Autodesk Fusion 360 part; units mm, degrees
sketch "Sketch1" plane through (0, 0, 0) normal (0, 1, 0) x (1, 0, 0)
  line L0 (0, 0) -> (0, -1175.3412)
  line L1 (0, -1175.3412) -> (0, 325) construction
  line L2 (0, 0) -> (-1356.5029, 0) construction
  circle A0 centre (871.6879, -79.2241) radius 125
  circle A1 centre (871.6879, -79.2241) radius 250
  line L3 (-50, 255) -> (50, 255)
  line L4 (50, 321.1308) -> (50, 933.0127)
  line L5 (-50, 945) -> (-50, 255)
  line L6 (250, 433.0127) -> (250, 933.0127)
  line L7 (-250, 933.0127) -> (-250, 433.0127)
  line L8 (635.6485, 3.1495) -> (499.9901, 3.1495)
  line L9 (490.5883, -96.5563) -> (622.2894, -96.5563)
  line L10 (-1356.5029, 0) -> (466.5356, 0) construction
  line L11 (634.5728, 0) -> (675.4964, 0) construction
  line L12 (775, 0) -> (1559.7574, 0) construction
  line L13 (250, 933.0127) -> (48.2627, 933.0127)
  line L14 (-48.2627, 933.0127) -> (-250, 933.0127)
  line L15 (-48.2627, 933.0127) -> (-50, 945) construction
  arc A2 (-250, 433.0127) -> (250, 433.0127) centre (0, 0) ccw
  arc A3 (-50, 321.1308) -> (50, 321.1308) centre (0, 0) ccw
  line L16 (99.0099, -490.099) -> (909.823, -326.2984)
  dimension "d1" = 650
  dimension "d2" = 1000
  dimension "d3" = 250
  dimension "d4" = 500
  dimension "d7" = 500
  dimension "d8" = 500
  dimension "d9" = 933.0127
extrude "Extrude1" add sketch "Sketch1" along normal mid plane 400 contours L0 L4 L6 L13 A2 A3 | L0 L5 L7 L14 A2 A3 | A1 L8 L9 A2 | A1
extrude "Extrude2" add sketch "Sketch1" along normal mid plane 100 contours A1 L9 A2 L16
hole "Hole1" at (250, 0, -683.0127) direction (-1, 0, 0) diameter 200 end through all
Geometry check sheet. Reference: the model listing, model coordinates, mm. A direction names the side the tool comes from. Round coordinates to 2 decimals unless told otherwise and drop trailing zeros. Loops run counter-clockwise (first coordinate to the right, second up) from the corner with the lowest first, then second, coordinate; pieces in that order, holes last.
Item 1: Cross-section at D-D on z = -764. Record the boundary of the cut face in (x, y), then the cut area to 3 significant figures.
Item 2: Cross-section at C-C on x = 545. Record the boundary of the cut face in (y, z), then the cut area to 3 significant figures.
Item 3: Cross-section at B-B on z = -559.5. Record the boundary of the cut face in (x, y).
Item 4: Mould release check, pull along Z, two halves, no side actions. Record for faces 1 (the cylindrical face through (1083.36, -2.8, -53.8)), 2 (the cylindrical face through (430.38, -2.8, -254.505)), 3 (the cylindrical face through (-151.4, -4.4, -583.11)): pulls with the +Z half, pulls with the -Z half, needs draft (parallel to the pull), parting line crosses it, or undercut.
Item 5: Cross-section at A-A on y = 0. Record the boundary of the cut face in (x, z), then the cut area to 3 significant figures.
Item 6: Access from +Z, -Z, +X, -X, +Y, -Y to the whole of each face (thin tool, end or side, straight path). Record for faces 4 (the flat face through (556, -126, 96.556)), 5 (the flat face through (569, -3, -3.15)), 6 (the flat face through (556, 124, 96.556)), 7 (the flat face through (250, -92, -735)).
Item 7: Thickness scan on line 1 (X direction, y = 136, z = 4.5); line 2 (Z direction, x = -144, y = 0); line 3 (X direction, y = -144, z = -685.5). Record the ranges inside material, lowest first.
Item 8: Gauge pin test, flat ends, axial feed: pin 1 (12 mm diameter, centred on x = 737.5, y = 114.5, fed in from -Z); pin 2 (12 mm diameter, centred on x = 521, y = 38, fed in from -Z); pin 3 (8 mm diameter, centred on x = 953, y = 98.5, fed in from -Z). Record the tip position at first contact, or that the pin passes through.
Answer sheet:
1. outline: (-250, -200) - (-50, -200) - (-50, -58.66) - (-250, -58.66) - close; (-250, 58.66) - (-50, 58.66) - (-50, 200) - (-250, 200) - close; (50, -200) - (250, -200) - (250, -58.66) - (50, -58.66) - close; (50, 58.66) - (250, 58.66) - (250, 200) - (50, 200) - close
1. area: 113,000 mm2
2. outline: (-200, -3.15) - (200, -3.15) - (200, 96.56) - (50, 96.56) - (50, 400) - (-50, 400) - (-50, 96.56) - (-200, 96.56) - close
2. area: 70,200 mm2
3. outline: (-250, -200) - (-50, -200) - (-50, 200) - (-250, 200) - close; (50, -200) - (250, -200) - (250, 200) - (50, 200) - close
4. face 1: parting line crosses it
4. face 2: pulls with the -Z half
4. face 3: undercut
5. outline: (-250, -933.01) - (-50, -933.01) - (-50, -783.01) - (-250, -783.01) - close; (-250, -583.01) - (-50, -583.01) - (-50, -321.13) arc R325 cw (long way) to (50, -321.13) - (50, -583.01) - (250, -583.01) - (250, -433.01) arc R500 ccw to (499.99, -3.15) - (635.65, -3.15) arc R250 ccw (long way) to (909.82, 326.3) - (99.01, 490.1) arc R500 ccw to (-250, -433.01) - close; (50, -933.01) - (250, -933.01) - (250, -783.01) - (50, -783.01) - close; hole circle Ø250 at (871.69, 79.22)
5. area: 790,000 mm2
6. face 4: +Z, -Y
6. face 5: -Z, +Y, -Y
6. face 6: +Z, +Y
6. face 7: -Z, +X, +Y, -Y
7. line 1: x = -499.98 to -324.97, 324.97 to 771.48, 971.89 to 1110.26
7. line 2: z = -933.01 to -783.01, -583.01 to -291.36, 291.36 to 478.82
7. line 3: x = -250 to -50, 50 to 250
8. pin 1: stops at z = -135.41
8. pin 2: stops at z = -3.15
8. pin 3: stops at z = -158.52
